Drawing for the job (mm, zero at the part's lowest x, y, z). Round coordinates to 2 decimals unless told otherwise and drop trailing zeros. Write each loop counter-clockwise with the first axis right and the second up, starting at its lowest first coordinate (ties: lowest second). Pieces come first, ordered by that corner, then holes. Notation, with made-up numbers: (-25.5, 7) -> (29.5, 7) arc R10 cw to (29.5, 22) -> close; hole circle Ø7 at (41, 53). An arc over 180 degrees is marked (long way). One line per question, with ' | ' between items.
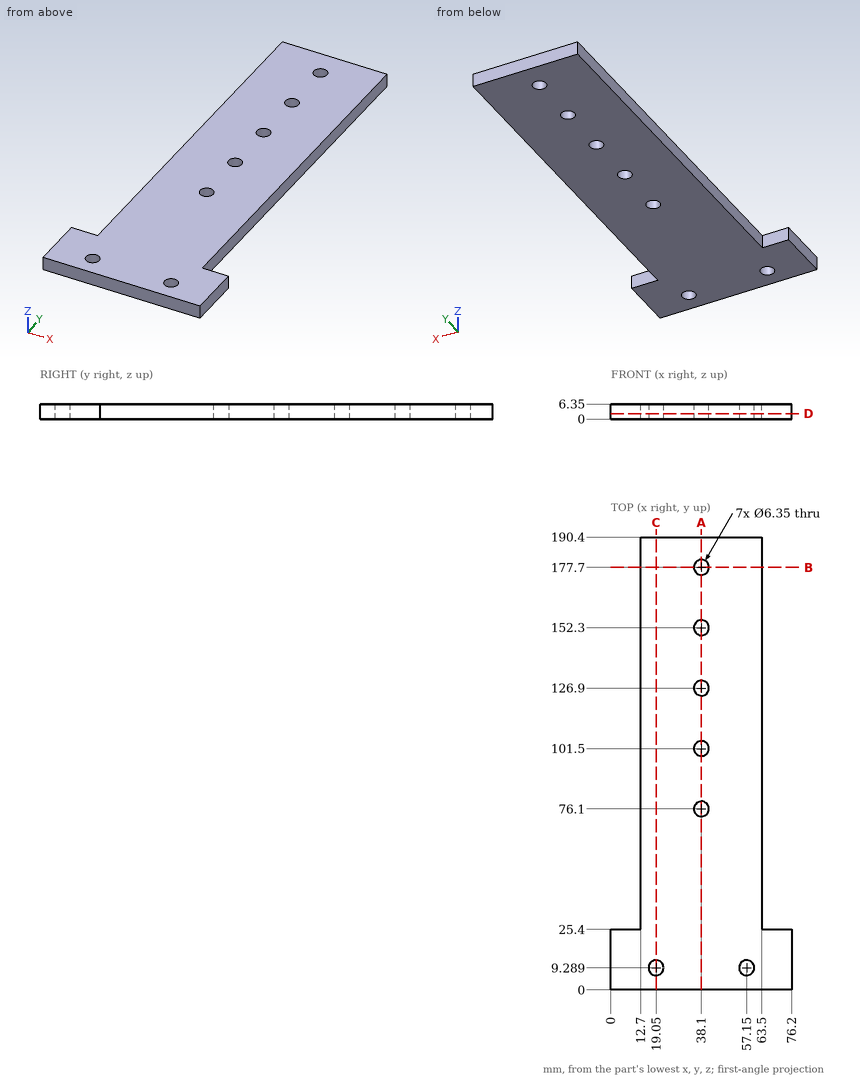
(1) Slice it at B-B (y = 177.7). Write the cut outline in (x, z) (3 decimals).
Calculated:
outline: (12.7, 0) -> (34.925, 0) -> (34.925, 6.35) -> (12.7, 6.35) -> close; (41.275, 0) -> (63.5, 0) -> (63.5, 6.35) -> (41.275, 6.35) -> close
(2) Slice it at D-D (z = 2.25). Write the cut outline in (x, y) (3 decimals), then the cut area to 3 significant figures.
Calculated:
outline: (0, 0) -> (76.2, 0) -> (76.2, 25.4) -> (63.5, 25.4) -> (63.5, 190.4) -> (12.7, 190.4) -> (12.7, 25.4) -> (0, 25.4) -> close; hole circle Ø6.35 at (19.05, 9.289); hole circle Ø6.35 at (38.1, 76.1); hole circle Ø6.35 at (38.1, 101.5); hole circle Ø6.35 at (38.1, 126.9); hole circle Ø6.35 at (38.1, 152.3); hole circle Ø6.35 at (38.1, 177.7); hole circle Ø6.35 at (57.15, 9.289) | area: 10,100 mm2
(3) Slice it at C-C (x = 19.05). Write the cut outline in (y, z).
Calculated:
outline: (0, 0) -> (6.11, 0) -> (6.11, 6.35) -> (0, 6.35) -> close; (12.46, 0) -> (190.4, 0) -> (190.4, 6.35) -> (12.46, 6.35) -> close
(4) Drop a flat-ended pin along its axis: pin 1 (5 mm diameter, centred on x = 19.05, y = 9.29, fed in from +Z). Give the stop position or say it passes through.
Calculated:
pin 1: through
(5) Wall check: line 1 (Y direction, x = 38.1, z = 2.5) (3 decimals); line 2 (Y direction, x = 57.15, z = 3); line 3 (Y direction, x = 6, z = 0.75). Give the ranges that are in metal, low to high. Write a range as from..to.
Calculated:
line 1: 0..72.925, 79.275..98.325, 104.675..123.725, 130.075..149.125, 155.475..174.525, 180.875..190.4 | line 2: 0..6.11, 12.46..190.4 | line 3: 0..25.4
(6) Slice it at A-A (x = 38.1). Write the cut outline in (y, z) (3 decimals).
Calculated:
outline: (0, 0) -> (72.925, 0) -> (72.925, 6.35) -> (0, 6.35) -> close; (79.275, 0) -> (98.325, 0) -> (98.325, 6.35) -> (79.275, 6.35) -> close; (104.675, 0) -> (123.725, 0) -> (123.725, 6.35) -> (104.675, 6.35) -> close; (130.075, 0) -> (149.125, 0) -> (149.125, 6.35) -> (130.075, 6.35) -> close; (155.475, 0) -> (174.525, 0) -> (174.525, 6.35) -> (155.475, 6.35) -> close; (180.875, 0) -> (190.4, 0) -> (190.4, 6.35) -> (180.875, 6.35) -> close
